from build123d import *

# Parameters (mm, degrees)
BOSS_EXTRUDE1_DEPTH = 2
SKETCH2_W           = 9
SKETCH2_H           = 9
BOSS_EXTRUDE2_DEPTH = 4.5


with BuildPart() as part:
    # Sketch1 → Boss-Extrude1 (new body)
    with BuildSketch(Plane(origin=(0, 0, 0), x_dir=(1, 0, 0), z_dir=(0, 1, 0))):
        with BuildLine():
            add(Edge.make_bspline(
                [(-6.730667633, 6.730667633), (-89.181346144, 0), (-6.730667633, -6.730667633)],
                knots=[4.990688639, 4.990688639, 4.990688639, 7.575681975, 7.575681975, 7.575681975], degree=2, weights=[1, 0.274721128, 1]))
            add(Edge.make_bspline(
                [(-6.730667633, -6.730667633), (0, -89.181346144), (6.730667633, -6.730667633)],
                knots=[4.990688639, 4.990688639, 4.990688639, 7.575681975, 7.575681975, 7.575681975], degree=2, weights=[1, 0.274721128, 1]))
            add(Edge.make_bspline(
                [(6.730667633, -6.730667633), (89.181346144, 0), (6.730667633, 6.730667633)],
                knots=[1.849095986, 1.849095986, 1.849095986, 4.434089321, 4.434089321, 4.434089321], degree=2, weights=[1, 0.274721128, 1]))
            add(Edge.make_bspline(
                [(6.730667633, 6.730667633), (0, 89.181346144), (-6.730667633, 6.730667633)],
                knots=[1.849095986, 1.849095986, 1.849095986, 4.434089321, 4.434089321, 4.434089321], degree=2, weights=[1, 0.274721128, 1]))
        make_face()
    extrude(amount=BOSS_EXTRUDE1_DEPTH)

    # Sketch2 → Boss-Extrude2 (add)
    with BuildSketch(Plane(origin=(0, 2, 0), x_dir=(1, 0, 0), z_dir=(0, 1, 0))):
        Rectangle(SKETCH2_W, SKETCH2_H)
    extrude(amount=BOSS_EXTRUDE2_DEPTH)


solid = part.part
CAD build for the part. Positions are in the model's coordinates, mm. A direction names the side the tool comes from. Round coordinates to 2 decimals unless told otherwise and drop trailing zeros. Write each loop counter-clockwise with the first axis right and the second up, starting at its lowest first coordinate (ties: lowest second). Pieces come first, ordered by that corner, then holes. Notation, with made-up numbers: M 63.5,81 L 104.5,81 A17 cw 104.5,101 Z; hole C 23,83 d2. An arc over 180 degrees is marked long. Use a Markdown table: item, result. Add a question column.
1. Drill centre lines: probe 1 along X at (y, z) = (2.75, 3); probe 2 along Y at (x, z) = (13, -3). Where is each one in solid material? Low to high.
2. Flat gauge pins, fed straight in: P1, Ø1, axis at x = 18, y = 4, coming from the +Z side; P2, Ø1.5, axis at x = -3, z = 10.5, coming from the +Y side; P3, Ø1.3, axis at x = -0.5, y = 3.5, coming from the +Z side; P4, Ø2, axis at y = 5.5, z = -0.5, coming from the +X side. Where does each tip first touch, or does it go through?
3. Slice it at A-A on y = 4.75. Give the cut face in (x, z).
4. 3-axis set-ups, long thin cutter, end or side, ignore diameter. For faces 1 (the face through (0, 4, -4.5)), 2 (the face through (0, 4, 4.5)), 3 (the face through (-4.5, 4, 0)), 4 (the face through (4.5, 4, 0)): which of +Z, -Z, +X, -X, +Y, -Y reach the whole face in a straight line?
Reply:
| question | item | result |
|---|---|---|
| 1 | probe 1 | x = -4.5 to 4.5 |
| 1 | probe 2 | y = 0 to 2 |
| 2 | P1 | passes through |
| 2 | P2 | stops at y = 2 |
| 2 | P3 | stops at z = 4.5 |
| 2 | P4 | stops at x = 4.5 |
| 3 | outline | M -4.5,-4.5 L 4.5,-4.5 L 4.5,4.5 L -4.5,4.5 Z |
| 4 | face 1 | -Z, +X, -X, +Y |
| 4 | face 2 | +Z, +X, -X, +Y |
| 4 | face 3 | +Z, -Z, -X, +Y |
| 4 | face 4 | +Z, -Z, +X, +Y |
